Read the model definition and answer for the solid it produces. Units are mm, in the model's axes. A direction names the side the tool comes from. Coordinates: 2 decimals unless noted, no trailing zeros. Order: outer loops, then holes, each group sorted by start corner. A loop starts at its lowest first (then second) coordinate and runs counter-clockwise, first axis right, second up. Notation, with made-up numbers: M -19.75,78.25 L 29.25,78.25 A4 cw 29.25,83.25 Z; hole C -38,-6 d9. An arc over 180 degrees is marked long. Put each result on its own line as item: value.
Autodesk Inventor part; units mm, degrees
ref_plane "YZ Plane" through (0, 0, 0) normal (1, 0, 0) x (0, 1, 0)
ref_plane "XZ Plane" through (0, 0, 0) normal (0, 1, 0) x (-1, 0, 0)
ref_plane "XY Plane" through (0, 0, 0) normal (0, 0, 1) x (1, 0, 0)
ref_plane "Work Plane1" through (-27.4782, 47.3, -1.2107) normal (0.118263, 0, 0.9929823) x (0, -1, 0)
sketch "Sketch1" plane through (-27.4782, 47.3, -1.2107) normal (0.118263, 0, 0.9929823) x (0, -1, 0)
  line L0 (0, 33.4421) -> (0, -8.2516)
  line L1 (2, -10.2376) -> (92.6, -10.2376)
  line L2 (94.6, -8.2516) -> (94.6, 33.4421)
  line L3 (92.6, 35.428) -> (2, 35.428)
  line L4 (7, -3.2867) -> (7, 28.4771)
  line L5 (7, 28.4771) -> (87.6, 28.4771)
  line L6 (87.6, 28.4771) -> (87.6, -3.2867)
  line L7 (87.6, -3.2867) -> (7, -3.2867)
  ellipse E0 centre (2, 33.4421) end of major axis (4, 33.4421) minor radius 1.986 (2, 35.428) -> (0, 33.4421) ccw
  ellipse E1 centre (2, -8.2516) end of major axis (0, -8.2516) minor radius 1.986 (0, -8.2516) -> (2, -10.2376) ccw
  ellipse E2 centre (92.6, -8.2516) end of major axis (90.6, -8.2516) minor radius 1.986 (92.6, -10.2376) -> (94.6, -8.2516) ccw
  ellipse E3 centre (92.6, 33.4421) end of major axis (94.6, 33.4421) minor radius 1.986 (94.6, 33.4421) -> (92.6, 35.428) ccw
  ellipse E4 centre (91.1, -6.7621) end of major axis (92.6, -6.7621) minor radius 1.4895
  ellipse E5 centre (3.5, -6.7621) end of major axis (5, -6.7621) minor radius 1.4895
  ellipse E6 centre (91.1, 31.9526) end of major axis (92.6, 31.9526) minor radius 1.4895
  ellipse E7 centre (3.5, 31.9526) end of major axis (5, 31.9526) minor radius 1.4895
  point P0 (47.3, 27.1422)
extrude "Extrusion1" add sketch "Sketch1" along normal blind 5 contours E0 L3 E3 L2 E2 L1 E1 L0 | L4 L5 L6 L7
sketch "Sketch2" plane through (-26.8869, 47.3, 3.7542) normal (0.118263, 0, 0.9929823) x (0.9929823, 0, -0.118263)
  line L0 (16.6422, -25.3) -> (37.6422, -25.3)
  line L1 (37.6422, -25.3) -> (37.6422, -69.3)
  line L2 (37.6422, -69.3) -> (16.6422, -69.3)
  line L3 (16.6422, -69.3) -> (16.6422, -25.3)
  line L4 (16.6422, -25.3) -> (37.6422, -69.3) construction
  line L5 (37.6422, -25.3) -> (16.6422, -69.3) construction
  line L6 (37.6422, -27.8) -> (16.6422, -27.8)
  arc A0 (37.6422, -27.8) -> (16.6422, -27.8) centre (27.1422, -48.6) ccw
  line L7 (33.4421, 0) -> (-8.2516, 0)
  arc A1 (-8.2516, 0) -> (-10.2376, -2) centre (2, -2) ccw
  line L8 (-10.2376, -2) -> (-10.2376, -92.6)
  arc A2 (-10.2376, -92.6) -> (-8.2516, -94.6) centre (2, -92.6) ccw
  line L9 (-8.2516, -94.6) -> (33.4421, -94.6)
  arc A3 (33.4421, -94.6) -> (35.428, -92.6) centre (45.9099, -92.6) ccw
  line L10 (35.428, -92.6) -> (35.428, -2)
  arc A4 (35.428, -2) -> (33.4421, 0) centre (45.9099, -2) ccw
  circle A5 centre (44.4099, -3.5) radius 1.5
  circle A6 centre (44.4099, -91.1) radius 1.5
  circle A7 centre (3.5, -3.5) radius 1.5
  circle A8 centre (3.5, -91.1) radius 1.5
  line L11 (35.428, -47.3) -> (-10.2376, -47.3)
  line L12 (-10.2376, -2) -> (-10.2376, -92.6)
  arc A9 (16.6422, -66.8) -> (37.6422, -66.8) centre (27.1422, -46) ccw
  point P0 (27.1422, -47.3)
  point P1 (27.1422, -25.3)
  point P2 (16.6422, -66.8)
  point P3 (37.6422, -66.8)
  dimension "d2" = 21
  dimension "d3" = 44
  dimension "d4" = 2.5
extrude "Extrusion2" cut sketch "Sketch2" against normal through all contours A0 L10 L6 | L6 L10 L11 L3 | A0 L6 L10 | L11 L10 A9 L3 | L6 L1 A9 L10
sketch "Sketch3" plane through (-27.4782, 47.3, -1.2107) normal (-0.118263, 0, -0.9929823) x (-0.9929823, 0, 0.118263)
  arc A0 (-35.428, -67.7769) -> (-16.6422, -66.8) centre (-27.1422, -46) ccw
  arc A1 (-16.6422, -27.8) -> (-35.428, -26.8231) centre (-27.1422, -48.6) ccw
  line L0 (-16.6422, -27.8) -> (-16.6422, -66.8)
  line L1 (-33.4421, 0) -> (8.2516, 0)
  arc A2 (-33.4421, 0) -> (-35.428, -2) centre (-45.9099, -2) ccw
  line L2 (-35.428, -92.6) -> (-35.428, -67.7769)
  arc A3 (-35.428, -92.6) -> (-33.4421, -94.6) centre (-45.9099, -92.6) ccw
  line L3 (8.2516, -94.6) -> (-33.4421, -94.6)
  arc A4 (8.2516, -94.6) -> (10.2376, -92.6) centre (-2, -92.6) ccw
  line L4 (10.2376, -2) -> (10.2376, -92.6)
  arc A5 (10.2376, -2) -> (8.2516, 0) centre (-2, -2) ccw
  circle A6 centre (-44.4099, -3.5) radius 1.5
  circle A7 centre (-44.4099, -91.1) radius 1.5
  circle A8 centre (-3.5, -3.5) radius 1.5
  circle A9 centre (-3.5, -91.1) radius 1.5
  line L5 (-6.7624, 0) -> (0.2376, 0)
  line L6 (0.2376, 0) -> (0.2376, -12.0472)
  line L7 (-1.7624, -14.0472) -> (-4.7624, -14.0472)
  line L8 (-6.7624, -12.0472) -> (-6.7624, 0)
  arc A10 (-6.7624, -12.0472) -> (-4.7624, -14.0472) centre (-4.7624, -12.0472) ccw
  arc A11 (-1.7624, -14.0472) -> (0.2376, -12.0472) centre (-1.7624, -12.0472) ccw
  line L9 (0.2376, -7) -> (-6.7624, -7)
  line L10 (-35.428, -26.8231) -> (-35.428, -2)
  point P0 (-27.1422, -47.3)
  point P1 (0.2376, -14.0472)
  point P2 (-6.7624, -14.0472)
  point P3 (0.2376, 0)
  dimension "d7" = 7
  dimension "d9" = 2
  dimension "d12" = 10
  dimension "d13" = 7
extrude "Extrusion3" cut sketch "Sketch3" against normal through all contours L1 L6 L9 L8 | L9 L6 A11 L7 A10 L8 | A8
properties part number "TAPA_CAMARA_2"
Q1. Given pin 1 (1.1 mm diameter, centred on x = -24.5, z = 1, fed in from +Y); pin 2 (1.5 mm diameter, centred on x = -20.5, y = -34.5, fed in from -Z), each flat-ended and moving along its own axis, determine where each tip first touches the part or whether it passes through.
Answers below:
pin 1: stops at y = 33.25
pin 2: stops at z = -2.13
Q2. A tool of negligible diameter and unlimited length cuts with its end or side. For faces 4 (the face through (-20.47, 41.19, 0.44)), 5 (the face through (-26.8, 33.8, 1.2)), 6 (the face through (-1.294, 21.975, -1.776)), from which of +Z, -Z, +X, -X, +Y, -Y can it reach the whole face along a straight path? Write none if from no direction.
Answers below:
face 4: +Z, +Y
face 5: -Z, +Y
face 6: none
Q3. Consider line 1 along Y through (x, z) = (-1.5, -3.75); line 2 along Z through (x, y) = (-24.5, 22.5); line 3 along Z through (x, y) = (5, -23). Determine where each line is inside the solid, lowest interval first.
Answers below:
line 1: y = -47.3 to -21.98, 21.98 to 47.3
line 2: z = -1.57 to 3.47
line 3: z = -5.08 to -0.04
Q4. Find section A-A on y = -16. Write down the section's boundary in (x, z), plus the area to 3 significant figures.
Answers below:
outline: M -37.64,0 L -10.95,-3.18 L -10.36,1.79 L -37.05,4.96 Z
area: 134 mm^2
Q5. Find section B-B on x = -17.5. Write down the section's boundary in (y, z), plus the area to 3 significant figures.
Answers below:
outline: M -47.3,-2.4 L 47.3,-2.4 L 47.3,2.64 L -47.3,2.64 Z
area: 476 mm^2
Q6. For a pull along X with two mould halves and no side action, classify faces 1 (the face through (-37.352, 0.634, 2.448)), 2 (the face through (-27.423, 41.361, 1.265)), 3 (the face through (-10.653, -0.273, -0.662)) as +X half, -X half, draft (parallel to the pull), parting line (faces both ways), or undercut.
Answers below:
face 1: -X half
face 2: undercut
face 3: +X half
